For this review, take the finished solid that the model builds, in its own axes (mm). Give positions to 0.01 mm unless a question says otherwise; leave off trailing zeros. Order: outer loops, then holes, each group sorted by start corner. A loop starts at its lowest first (then second) coordinate and runs counter-clockwise, first axis right, second up.
Item 1: For probe 1 along X at (y, z) = (1.4, 0); probe 2 along X at (y, z) = (1.2, 80); probe 3 along Z at (x, y) = (39, 0.3), list the stretches that pass through material, from the lowest coordinate up.
Item 2: Consider section A-A (z = 54). Give the boundary of the cut face in (x, y).
Item 3: Consider section C-C (z = 0). Give the boundary of the cut face in (x, y), plus the area to 3 significant figures.
Item 4: Consider section D-D (x = 37). Give the boundary of the cut face in (y, z).
Item 5: Consider section B-B (x = -90). Give the boundary of the cut face in (y, z).
```python
from build123d import *

# Parameters (mm, degrees)
SKETCH_1_W      = 215
SKETCH_1_H      = 190
SKETCH_1_R      = 4.4
SKETCH_1_W_2    = 145
SKETCH_1_H_2    = 120
EXTRUDE_1_DEPTH = 2
FILLET_1_R      = 10


with BuildPart() as part:
    # Эскиз1 → Бобышка-Вытянуть1 (new body)
    with BuildSketch(Plane(origin=(0, 0, 0), x_dir=(1, 0, 0), z_dir=(0, 1, 0))):
        Rectangle(SKETCH_1_W, SKETCH_1_H)
        with Locations(Location((-90, 80, 0), (0, 0, 270))):
            Circle(SKETCH_1_R, mode=Mode.SUBTRACT)
        with Locations(Location((-90, -80, 0), (0, 0, 90))):
            Circle(SKETCH_1_R, mode=Mode.SUBTRACT)
        with Locations(Location((-90, 0, 0), (0, 0, 270))):
            Circle(SKETCH_1_R, mode=Mode.SUBTRACT)
        with Locations(Location((-30, -80, 0), (0, 0, 90))):
            Circle(SKETCH_1_R, mode=Mode.SUBTRACT)
        with Locations(Location((-30, 80, 0), (0, 0, 270))):
            Circle(SKETCH_1_R, mode=Mode.SUBTRACT)
        with Locations(Location((30, -80, 0), (0, 0, 90))):
            Circle(SKETCH_1_R, mode=Mode.SUBTRACT)
        with Locations(Location((30, 80, 0), (0, 0, 270))):
            Circle(SKETCH_1_R, mode=Mode.SUBTRACT)
        with Locations(Location((90, -80, 0), (0, 0, 90))):
            Circle(SKETCH_1_R, mode=Mode.SUBTRACT)
        with Locations(Location((90, 0, 0), (0, 0, 270))):
            Circle(SKETCH_1_R, mode=Mode.SUBTRACT)
        with Locations(Location((90, 80, 0), (0, 0, 270))):
            Circle(SKETCH_1_R, mode=Mode.SUBTRACT)
        Rectangle(SKETCH_1_W_2, SKETCH_1_H_2, mode=Mode.SUBTRACT)
    extrude(amount=EXTRUDE_1_DEPTH)

    # Скругление1
    fillet_1_edges = [part.edges().sort_by_distance(p)[0] for p in [
        (107.5, 1, -95),
        (107.5, 1, 95),
        (-107.5, 1, 95),
        (-107.5, 1, -95),
    ]]
    fillet(fillet_1_edges, radius=FILLET_1_R)


solid = part.part
```
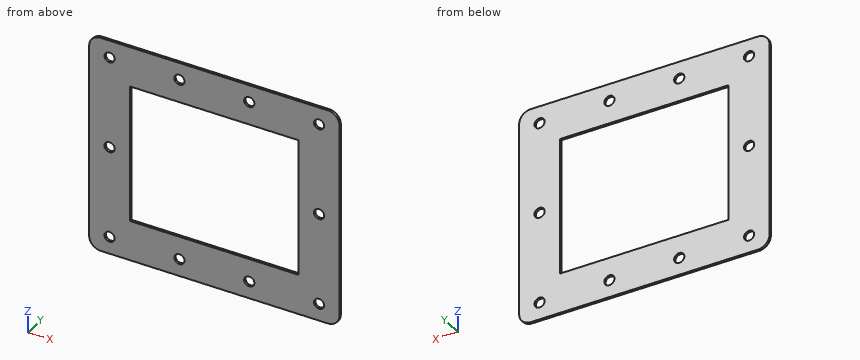
Resolved:
1. probe 1: x = -107.5 to -94.4, -85.6 to -72.5, 72.5 to 85.6, 94.4 to 107.5
1. probe 2: x = -107.5 to -94.4, -85.6 to -34.4, -25.6 to 25.6, 34.4 to 85.6, 94.4 to 107.5
1. probe 3: z = -95 to -60, 60 to 95
2. outline: (-107.5, 0) - (-72.5, 0) - (-72.5, 2) - (-107.5, 2) - close; (72.5, 0) - (107.5, 0) - (107.5, 2) - (72.5, 2) - close
3. outline: (-107.5, 0) - (-94.4, 0) - (-94.4, 2) - (-107.5, 2) - close; (-85.6, 0) - (-72.5, 0) - (-72.5, 2) - (-85.6, 2) - close; (72.5, 0) - (85.6, 0) - (85.6, 2) - (72.5, 2) - close; (94.4, 0) - (107.5, 0) - (107.5, 2) - (94.4, 2) - close
3. area: 105 mm2
4. outline: (0, -95) - (2, -95) - (2, -60) - (0, -60) - close; (0, 60) - (2, 60) - (2, 95) - (0, 95) - close
5. outline: (0, -95) - (2, -95) - (2, -84.4) - (0, -84.4) - close; (0, -75.6) - (2, -75.6) - (2, -4.4) - (0, -4.4) - close; (0, 4.4) - (2, 4.4) - (2, 75.6) - (0, 75.6) - close; (0, 84.4) - (2, 84.4) - (2, 95) - (0, 95) - close
